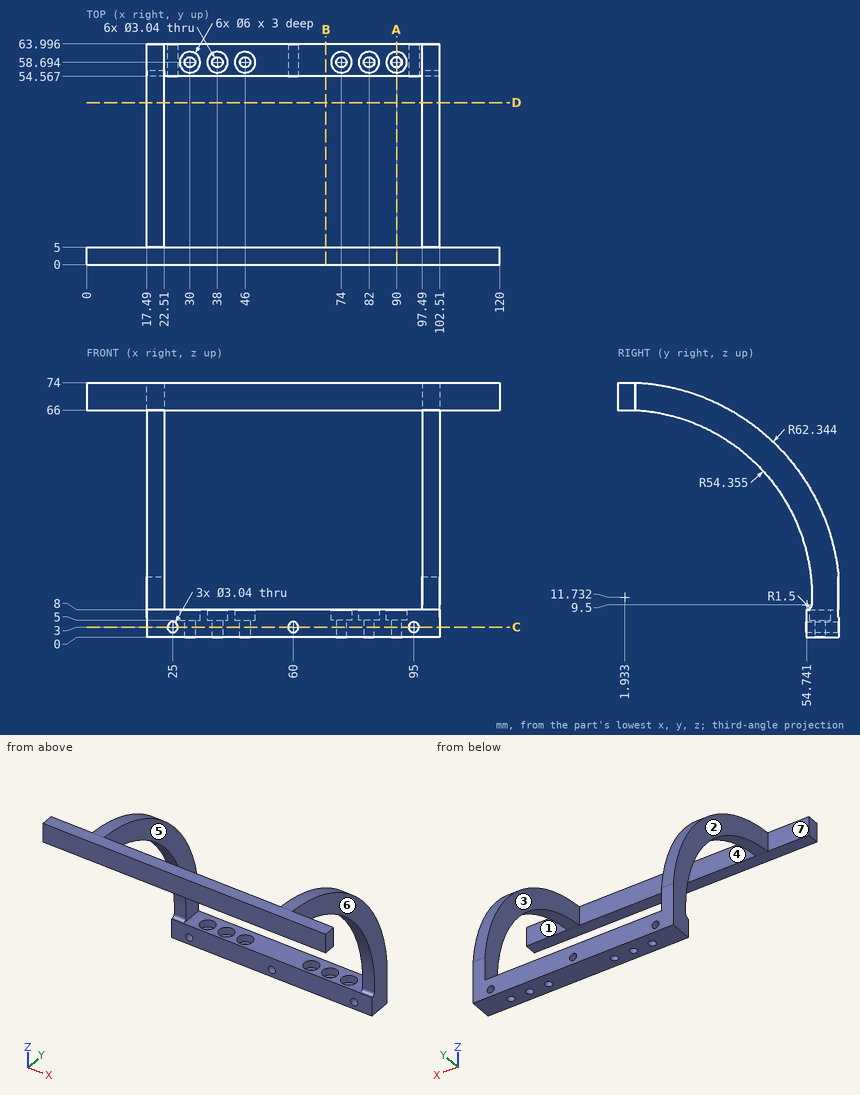
Here's the drawing with two shaded views (mm, measured from the low corner). I have some questions. A direction names the side the tool comes from. Round coordinates to 2 decimals unless told otherwise and drop trailing zeros. Loops run counter-clockwise (first coordinate to the right, second up) from the corner with the lowest first, then second, coordinate; pieces in that order, holes last. Notation, with made-up numbers: (77.25, 86) -> (117.25, 86) arc R15 cw to (117.25, 108) -> close; hole circle Ø10 at (55.5, 39). An arc over 180 degrees is marked (long way). Answer as CSV lines item,"result". Start each with the question number.
1. Imagine slicing it at B-B on x = 69.5. Write out the boundary of the cut face in (y, z) (1 decimal), plus the area to 3 significant figures.
2. Imagine slicing it at C-C on z = 3. State how many separate pieces and enclosed holes the cut face has, plus the area to 3 significant figures.
3. For the marked faces 1, 2, 3 and 4, which set-ups out of +Z, -Z, +X, -X, +Y, -Y let a thin tool reach every point of the face, with its end or its side?
4. I'm going to push flat-ended pins straight in: P1, Ø6, axis at y = 34.5, z = 57.5, coming from the +X side; P2, Ø1.5, axis at y = 22, z = 65, coming from the -X side; P3, Ø4, axis at x = 98.5, z = 29, coming from the +Y side; P4, Ø17.5, axis at y = 30.5, z = 36.5, coming from the -X side. Where does each tip first touch, or does it pass through?
5. Imagine slicing it at D-D on y = 47. Write out the boundary of the cut face in (x, z), plus the area to 3 significant figures.
6. If we mould it in two halves opening along X, with no side actions, what happens to the marked faces 5, 6 and 7? For each: pulls with the +X half, pulls with the -X half, needs draft (parallel to the pull), parting line crosses it, or undercut.
7. Imagine slicing it at A-A on x = 90. Write out the boundary of the cut face in (y, z) (1 decimal).
8. I need wall thicknesses on probe 1 along X at (y, z) = (56.5, 23); probe 2 along Y at (x, z) = (90, 5.95) (1 decimal); probe 3 along Y at (x, z) = (30, 2.2) (1 decimal). Which ranges of each line are inside material? Lowest first, please. Write a range as from..to.
Solution:
1,outline,"(0, 66) -> (5, 66) -> (5, 74) -> (0, 74) -> close; (54.6, 0) -> (64, 0) -> (64, 8) -> (54.6, 8) -> close"
1,area,"115 mm²"
2,separate pieces,"4"
2,enclosed holes,"6"
2,area,"672 mm²"
3,face 1,"+Z, -Z, +X, +Y"
3,face 2,"+Z, -Z, -X, +Y"
3,face 3,"+Z, +Y"
3,face 4,"+Z, -Z, +Y"
4,P1,"x = 102.51"
4,P2,"x = 17.49"
4,P3,"y = 62.38"
4,P4,"through"
5,outline,"(17.49, 42.12) -> (22.51, 42.12) -> (22.51, 54.81) -> (17.49, 54.81) -> close; (97.49, 42.12) -> (102.51, 42.12) -> (102.51, 54.81) -> (97.49, 54.81) -> close"
5,area,"127 mm²"
6,face 5,"undercut"
6,face 6,"pulls with the +X half"
6,face 7,"needs draft"
7,outline,"(0, 66) -> (5, 66) -> (5, 74) -> (0, 74) -> close; (54.6, 0) -> (57.2, 0) -> (57.2, 5) -> (55.7, 5) -> (55.7, 8) -> (54.6, 8) -> close; (60.2, 0) -> (64, 0) -> (64, 8) -> (61.7, 8) -> (61.7, 5) -> (60.2, 5) -> close"
8,probe 1,"17.49..22.51, 97.49..102.51"
8,probe 2,"54.6..55.7, 61.7..64"
8,probe 3,"54.6..57.2, 60.2..64"
